```python
from build123d import *

# Parameters (mm, degrees)
SKETCH1_R           = 12.5
BOSS_EXTRUDE1_DEPTH = 60
SKETCH2_R           = 5.6
BOSS_EXTRUDE2_DEPTH = 5


with BuildPart() as part:
    # Sketch1 → Boss-Extrude1 (new body)
    with BuildSketch(Plane(origin=(0, 0, 0), x_dir=(0, 0, -1), z_dir=(1, 0, 0))):
        with BuildLine():
            Line((-17.5, 0), (-17.5, 80))
            ThreePointArc((-17.5, 80), (-15, 82.5), (-12.5, 80))
            Line((-12.5, 80), (-12.5, 12.247448714))
            ThreePointArc((-12.5, 12.247448714), (16.201851746, -6.614378278), (-17.5, 0))
        make_face()
        Circle(SKETCH1_R, mode=Mode.SUBTRACT)
    extrude(amount=BOSS_EXTRUDE1_DEPTH)

    # Sketch2 → Boss-Extrude2 (add)
    with BuildSketch(Plane(origin=(0, 0, 0), x_dir=(0, 0, -1), z_dir=(1, 0, 0))):
        with BuildLine():
            ThreePointArc((2.5, 24.720508076), (11.1, 33.320508076), (2.5, 41.920508076))
            Line((2.5, 41.920508076), (-12.5, 41.920508076))
            Line((-12.5, 41.920508076), (-12.5, 12.247448714))
            ThreePointArc((-12.5, 12.247448714), (-5.606601718, 16.577575733), (2.5, 17.320508076))
            Line((2.5, 17.320508076), (2.5, 24.720508076))
        make_face()
        with Locations((2.5, 33.320508076)):
            Circle(SKETCH2_R, mode=Mode.SUBTRACT)
    extrude(amount=BOSS_EXTRUDE2_DEPTH)


solid = part.part
```
Can you work these out from the model? Positions are in its coordinate system, mm. A direction names the side the tool comes from. Give positions to 0.01 mm unless a question says otherwise; leave off trailing zeros. Loops run counter-clockwise (first coordinate to the right, second up) from the corner with the lowest first, then second, coordinate; pieces in that order, holes last. Notation, with made-up numbers: M 11.5,28.5 L 26.5,28.5 A18 ccw 26.5,47.5 Z; hole C 25,-25 d8. An arc over 180 degrees is marked long. One line per item, written item: value.
(1) Will these pins go through, and if not, where does the flat tip stop? pin 1 (1.5 mm diameter, centred on x = 2, z = 5.5, fed in from +Y); pin 2 (12 mm diameter, centred on x = 39, y = 37.5, fed in from -Z); pin 3 (1.5 mm diameter, centred on x = 37, z = -7.5, fed in from +Y).
Returned:
pin 1: y = 41.92
pin 2: z = 12.5
pin 3: y = 16.15
(2) Which directions (+Z, -Z, +X, -X, +Y, -Y) give clear straight access to the entire face, cutting with the end or side of a thin tool? Please do faces 4 (the face through (2, 21, -2.5)), 5 (the face through (2, 41.921, 5)), 6 (the face through (60, 25, 13)).
Returned:
face 4: -Z, +X, -X
face 5: -Z, +X, -X, +Y
face 6: +Z, -Z, +X, +Y, -Y
(3) We'd pull the mould along Y, two halves only. Please class faces 1 (the face through (29.6, 82.5, 15.1)), 2 (the face through (30, 47, 12.5)), 3 (the face through (2.465, 38.873, -1.771)): released by +Y, released by -Y, zero draft, split by the parting line, or undercut.
Returned:
face 1: released by +Y
face 2: zero draft
face 3: undercut
(4) Suppose I cut it at B-B on y = -8.5. List the corners of the cut face in (x, z) for me, plus the area to 3 significant figures.
Returned:
outline: M 0,-15.3 L 60,-15.3 L 60,-9.17 L 0,-9.17 Z; M 0,9.17 L 60,9.17 L 60,15.3 L 0,15.3 Z
area: 736 mm^2
(5) I need wall thicknesses on line 1 (Y direction, x = 16, z = 0); line 2 (Y direction, x = 3, z = -2); line 3 (Z direction, x = 36.5, y = 51). Which ranges of each line are inside material? Lowest first, please.
Returned:
line 1: -17.5 to -12.5, 12.5 to 17.5
line 2: -17.39 to -12.34, 12.34 to 27.74, 38.9 to 41.92
line 3: 12.5 to 17.5
(6) Suppose I cut it at A-A on x = 21. List the corners of the cut face in (y, z) for me, plus the area to 3 significant figures.
Returned:
outline: M 0,17.5 A17.5 ccw long 12.25,12.5 L 80,12.5 A2.5 ccw 80,17.5 Z; hole C 0,0 d25
area: 839 mm^2
(7) Suppose I cut it at D-D on y = 63. List the corners of the cut face in (x, z) for me, plus the area to 3 significant figures.
Returned:
outline: M 0,12.5 L 60,12.5 L 60,17.5 L 0,17.5 Z
area: 300 mm^2
(8) Suppose I cut it at C-C on z = 0. List the corners of the cut face in (x, y) for me, plus the area to 3 significant figures.
Returned:
outline: M 0,-17.5 L 60,-17.5 L 60,-12.5 L 0,-12.5 Z; M 0,12.5 L 60,12.5 L 60,17.5 L 5,17.5 L 5,28.31 L 0,28.31 Z; M 0,38.33 L 5,38.33 L 5,41.92 L 0,41.92 Z
area: 672 mm^2
